Here's how the part is built. I have some questions about the finished solid (model axes, mm). Face numbers are marked on the shaded views. A direction names the side the tool comes from. Give positions to 0.01 mm unless a question says otherwise; leave off trailing zeros. Loops run counter-clockwise (first coordinate to the right, second up) from the corner with the lowest first, then second, coordinate; pieces in that order, holes last. Notation, with made-up numbers: (-18, 18) - (16, 18) arc R7 ccw to (16, 26) - close; hole circle Ø6 at (-0.75, 23.25). An arc over 180 degrees is marked (long way). Use a Markdown table: item, result.
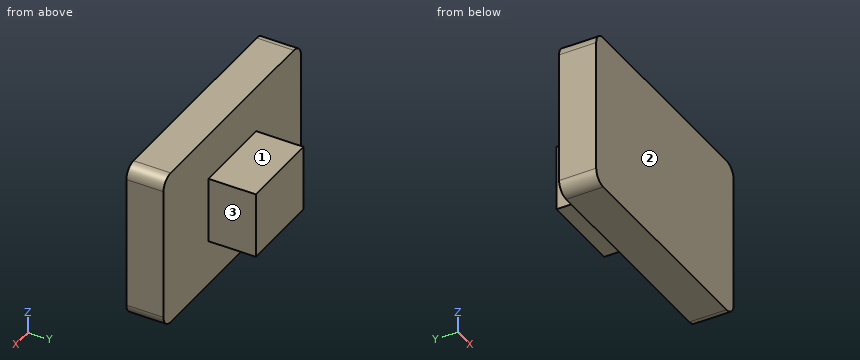
from build123d import *

# Parameters (mm, degrees)
EXTRUDE4_DEPTH = 19.05
SKETCH4_W      = 42.505133665
SKETCH4_H      = 33.908575234
EXTRUDE5_DEPTH = 24.384


with BuildPart() as part:
    # Sketch3 → Extrude4 (new body)
    with BuildSketch(Plane(origin=(0, 0, 0), x_dir=(1, 0, 0), z_dir=(0, 1, 0))):
        with BuildLine():
            Line((6.35, 0), (116.003921001, 0))
            ThreePointArc((116.003921001, 0), (120.494049062, 1.859871939), (122.353921001, 6.35))
            Line((122.353921001, 6.35), (122.353921001, 74.579258312))
            ThreePointArc((122.353921001, 74.579258312), (120.494049062, 79.069386372), (116.003921001, 80.929258312))
            Line((116.003921001, 80.929258312), (6.35, 80.929258312))
            ThreePointArc((6.35, 80.929258312), (1.859871939, 79.069386372), (0, 74.579258312))
            Line((0, 74.579258312), (0, 6.35))
            ThreePointArc((0, 6.35), (1.859871939, 1.859871939), (6.35, 0))
        make_face()
    extrude(amount=-EXTRUDE4_DEPTH)

    # Sketch4 → Extrude5 (add)
    with BuildSketch(Plane(origin=(0, 0, 0), x_dir=(1, 0, 0), z_dir=(0, 1, 0))):
        with Locations((61.176960501, 40.464629156)):
            Rectangle(SKETCH4_W, SKETCH4_H)
    extrude(amount=EXTRUDE5_DEPTH)


solid = part.part
(1) Suppose I cut it at D-D on z = -61.5. Write out the boundary of the cut face in (x, y), plus the area to 3 significant figures.
A:
| item | result |
|---|---|
| outline | (0, -19.05) - (122.35, -19.05) - (122.35, 0) - (0, 0) - close |
| area | 2,330 mm2 |
(2) Suppose I cut it at B-B on x = 78.5. Write out the boundary of the cut face in (y, z).
A:
| item | result |
|---|---|
| outline | (-19.05, -80.93) - (0, -80.93) - (0, -57.42) - (24.38, -57.42) - (24.38, -23.51) - (0, -23.51) - (0, 0) - (-19.05, 0) - close |
(3) On a 3-axis mill with a long thin cutter (end or side, diameter ignored), from which of +Z, -Z, +X, -X, +Y, -Y can I reach the whole of each face in a straight line? I mean the marked faces 1, 2 and 3. Say none if no direction works.
A:
| item | result |
|---|---|
| face 1 | +Z, +X, -X, +Y |
| face 2 | +Z, -Z, +X, -X, -Y |
| face 3 | +Z, -Z, +X, +Y |
(4) Suppose I cut it at C-C on y = 11.5. Write out the boundary of the cut face in (x, z).
A:
| item | result |
|---|---|
| outline | (39.92, -57.42) - (82.43, -57.42) - (82.43, -23.51) - (39.92, -23.51) - close |
(5) Will these pins go through, and if not, where does the flat tip stop? pin 1 (7.5 mm diameter, centred on x = 69, y = 10.5, fed in from +Z); pin 2 (3 mm diameter, centred on y = 17.5, z = -39, fed in from +X); pin 3 (4 mm diameter, centred on x = 61, z = -63.5, fed in from +Y).
A:
| item | result |
|---|---|
| pin 1 | z = -23.51 |
| pin 2 | x = 82.43 |
| pin 3 | y = 0 |
(6) If I drill on line 1 (X direction, y = 9, z = -34); line 2 (Y direction, x = 9, z = -62), over which ranges is the centre line in solid material (lowest first)?
A:
| item | result |
|---|---|
| line 1 | 39.92 to 82.43 |
| line 2 | -19.05 to 0 |
(7) Suppose I cut it at A-A on z = -37.5. Write out the boundary of the cut face in (x, y), plus the area to 3 significant figures.
A:
| item | result |
|---|---|
| outline | (0, -19.05) - (122.35, -19.05) - (122.35, 0) - (82.43, 0) - (82.43, 24.38) - (39.92, 24.38) - (39.92, 0) - (0, 0) - close |
| area | 3,370 mm2 |
